```python
from build123d import *

# Parameters (mm, degrees)
F1_DEPTH     = 38
F3_D         = 12
F4_R         = 10
F6_D         = 10
F8_DEPTH     = 2
F10_DEPTH    = 2
F11_W        = 30
F11_H        = 38
F12_DEPTH    = 2
F14_W        = 1
F14_H        = 15
F15_DEPTH    = 5
F16_W        = 2
F16_H        = 3
F18_DEPTH    = 2
F17_W        = 2
F17_H        = 3
F19_DEPTH    = 2
F20_SIZE     = 1.99999
F21_T1_DEPTH = 10.6602829052
F21_T3_DEPTH = 10.6602829052
F14_W_2      = 1.3
F14_H_2      = 15.3
F22_DEPTH    = 1


# Not quite as in the source:
# - a fillet or chamfer that OpenCascade refuses, or shapes differently, is made with other operations: its cross-section is extruded or revolved along the edge and cut away or added
# - a fillet or chamfer is up to 0.001 mm smaller than in the source, because OpenCascade refuses the exact size
# - a feature names something its author has since deleted; it is built from what else it names


with BuildPart() as f1:
    # F0 (on Front) → F1 (new body)
    with BuildSketch(Plane.XZ):
        with BuildLine():
            Line((-30, 90), (-32, 90))
            Line((-32, 90), (-32, 9.5))
            ThreePointArc((-32, 9.5), (-28.6317279836, 1.3682720164), (-20.5, -2))
            Line((-20.5, -2), (0, -2))
            Line((0, -2), (0, 0))
            Line((0, 0), (-20, 0))
            ThreePointArc((-20, 0), (-27.0710678119, 2.9289321881), (-30, 10))
            Line((-30, 10), (-30, 90))
        make_face()
    extrude(amount=F1_DEPTH)

    # F3 (through all)
    with Locations(Plane.XY):
        with Locations((5, -19)):
            Hole(F3_D / 2)

    # F4
    f4_edges = [f1.edges().sort_by_distance(p)[0] for p in [
        (-31, -38, 90),
        (-31, 0, 90),
    ]]
    fillet(f4_edges, radius=F4_R)

    # F6 (through all)
    with Locations(Plane.YZ.offset(-30)):
        with Locations((-19, 75)):
            Hole(F6_D / 2)

    # F7 (on face) → F8 (join)
    with BuildSketch(Plane.XZ.offset(38)):
        with BuildLine():
            Line((-20, 0), (0, 0))
            Line((0, 0), (0, 40))
            Line((0, 40), (-30, 40))
            Line((-30, 40), (-30, 10))
            ThreePointArc((-30, 10), (-27.0710678119, 2.9289321881), (-20, 0))
        make_face()
    extrude(amount=-F8_DEPTH)

    # F9 (on face) → F10 (join)
    with BuildSketch(Plane(origin=(0, 0, 0), x_dir=(-1, 0, 0), z_dir=(0, 1, 0))):
        with BuildLine():
            Line((0, 40), (0, 0))
            Line((0, 0), (20, 0))
            ThreePointArc((20, 0), (27.0710678119, 2.9289321881), (30, 10))
            Line((30, 10), (30, 40))
            Line((30, 40), (0, 40))
        make_face()
    extrude(amount=-F10_DEPTH)

    # F11 (on face) → F12 (join)
    with BuildSketch(Plane.XY.offset(40)):
        with Locations((-15, -19)):
            Rectangle(F11_W, F11_H)
    extrude(amount=-F12_DEPTH)

    # F13: union 

    # F14 (on face) → F15 (join)
    with BuildSketch(Plane.YZ):
        with Locations((-1, 7.5)):
            Rectangle(F14_W, F14_H)
    extrude(amount=F15_DEPTH)

    # F16 (on face) → F18 (join)
    with BuildSketch(Plane.XZ.offset(2)):
        with Locations((-6.5, 10.5)):
            Rectangle(F16_W, F16_H)
        Polygon((-5, 5), (-5, 6), (-5, 7), (-8, 7), (-8, 5), align=None)
        with Locations((-23.5, 10.5)):
            Rectangle(F16_W, F16_H)
        Polygon((-25, 7), (-25, 6), (-25, 5), (-22, 5), (-22, 7), align=None)
    extrude(amount=F18_DEPTH)

    # F17 (on face) → F19 (join)
    with BuildSketch(Plane(origin=(0, -36, 0), x_dir=(-1, 0, 0), z_dir=(0, 1, 0))):
        with Locations((6.5, 10.5)):
            Rectangle(F17_W, F17_H)
        Polygon((5, 7), (5, 6), (5, 5), (8, 5), (8, 7), align=None)
        Polygon((25, 5), (25, 6), (25, 7), (22, 7), (22, 5), align=None)
        with Locations((23.5, 10.5)):
            Rectangle(F17_W, F17_H)
    extrude(amount=F19_DEPTH)

    # F20 (size 2 in the source; OpenCascade refuses exactly that, so slightly less here)
    f20_edges = [f1.edges().sort_by_distance(p)[0] for p in [
        (-6.5, -34, 12),
        (-23.5, -34, 12),
        (-6.5, -4, 12),
        (-23.5, -4, 12),
    ]]
    chamfer(f20_edges, length=F20_SIZE)

    # F21: fillet of radius 2 on 4 edges, made by hand

    # F21_s2 → F21_t1 (cut)
    with BuildSketch(Plane.YZ.offset(-11.8301414526)):
        with BuildLine():
            ThreePointArc((-35.732056581, 9), (-34.732051581, 9.2679520792), (-34, 10.00001))
            Line((-34, 10.00001), (-34, 9))
            Line((-34, 9), (-35.732056581, 9))
        make_face()
        with BuildLine():
            ThreePointArc((-2.267943419, 9), (-3.267948419, 9.2679520792), (-4, 10.00001))
            Line((-4, 10.00001), (-4, 9))
            Line((-4, 9), (-2.267943419, 9))
        make_face()
    extrude(amount=F21_T1_DEPTH, mode=Mode.SUBTRACT)

    # F21_s4 → F21_t3 (cut)
    with BuildSketch(Plane.YZ.offset(-28.8301414526)):
        with BuildLine():
            ThreePointArc((-34, 10.00001), (-34.732051581, 9.2679520792), (-35.732056581, 9))
            Line((-35.732056581, 9), (-34, 9))
            Line((-34, 9), (-34, 10.00001))
        make_face()
        with BuildLine():
            ThreePointArc((-2.267943419, 9), (-3.267948419, 9.2679520792), (-4, 10.00001))
            Line((-4, 10.00001), (-4, 9))
            Line((-4, 9), (-2.267943419, 9))
        make_face()
    extrude(amount=F21_T3_DEPTH, mode=Mode.SUBTRACT)

    # F14 (on face) → F22 (join)
    with BuildSketch(Plane.YZ):
        with Locations((-37, 7.5)):
            Rectangle(F14_W_2, F14_H_2)
    extrude(amount=F22_DEPTH)


solid = f1.part
```
For this review, take the finished solid that the model builds, in its own axes (mm). A direction names the side the tool comes from. Round coordinates to 2 decimals unless told otherwise and drop trailing zeros. Write each loop counter-clockwise with the first axis right and the second up, starting at its lowest first coordinate (ties: lowest second). Pieces come first, ordered by that corner, then holes. Notation, with made-up numbers: (53.25, -39.75) - (68.25, -39.75) arc R27 cw to (68.25, -16.75) - close; hole circle Ø8 at (-16.5, 26). An arc over 180 degrees is marked (long way). Write each question's results on one line, items separated by ' | '.
Item 1: To check wall thickness, follow line 1 along Z through (x, y) = (-11, -28); line 2 along Y through (x, z) = (-3, 28); line 3 along X through (y, z) = (-9, 26). State the ranges of each line that lie inside material, in increasing order. Write a range as from..to.
Calculated:
line 1: z = -2..0, 38..40 | line 2: y = -38..-36, -2..0 | line 3: x = -32..-30
Item 2: For faces 4 (the face through (-1, -19, -1)), 5 (the face through (-25, -35, 6)), 6 (the face through (-7, -3, 11)), list the 3-axis set-ups (+Z, -Z, +X, -X, +Y, -Y) from which the entire face can be reached by the end or side of a thin tool; tool diameter is ignored.
Calculated:
face 4: -Z, +X | face 5: none | face 6: +X
Item 3: For pin 1 (1.6 mm diameter, centred on y = -34.5, z = 6.5, fed in from -X); pin 2 (2 mm diameter, centred on y = -2.5, z = 6, fed in from -X) (3 decimals); pin 3 (6 mm diameter, centred on x = -20, y = -20, fed in from +Z), all flat-tipped, find the tip position at first contact; note any pin that passes through.
Calculated:
pin 1: stops at x = -31.79 | pin 2: stops at x = -31.725 | pin 3: stops at z = 40
Item 4: Draft analysis for pull direction Y (two halves, no side actions). For faces 1 (the face through (-32, -19, 50)), 2 (the face through (-16, -38, 21)), 3 (the face through (-24, -3, 5)), state which applies: pulls with the +Y half, pulls with the -Y half, needs draft (parallel to the pull), parting line crosses it, or undercut.
Calculated:
face 1: needs draft | face 2: pulls with the -Y half | face 3: undercut
Item 5: Take a section at C-C on y = -19. State the section outline as (x, z) points, then the cut area to 3 significant figures.
Calculated:
outline: (-32, 9.5) arc R11.5 ccw to (-20.5, -2) - (-1, -2) - (-1, 0) - (-20, 0) arc R10 cw to (-30, 10) - (-30, 38) - (0, 38) - (0, 40) - (-30, 40) - (-30, 70) - (-32, 70) - close; (-32, 80) - (-30, 80) - (-30, 90) - (-32, 90) - close | area: 275 mm^2
Item 6: Take a section at A-A on z = 75. State the section outline as (x, y) points, then the cut area to 3 significant figures.
Calculated:
outline: (-32, -38) - (-30, -38) - (-30, -24) - (-32, -24) - close; (-32, -14) - (-30, -14) - (-30, 0) - (-32, 0) - close | area: 56.0 mm^2
Item 7: Take a section at B-B on x = -14.5. State the section outline as (y, z) points, then the cut area to 3 significant figures.
Calculated:
outline: (-38, -2) - (0, -2) - (0, 40) - (-38, 40) - close; hole (-36, 0) - (-2, 0) - (-2, 38) - (-36, 38) - close | area: 304 mm^2
Item 8: Take a section at D-D on z = 14. State the section outline as (x, y) points.
Calculated:
outline: (-32, -38) - (0, -38) - (0, -37.65) - (1, -37.65) - (1, -36.35) - (0, -36.35) - (0, -36) - (-30, -36) - (-30, -2) - (0, -2) - (0, -1.5) - (5, -1.5) - (5, -0.5) - (0, -0.5) - (0, 0) - (-32, 0) - close
